from build123d import *

# Parameters (mm, degrees)
SKETCH2_R           = 2.032
BOSS_EXTRUDE1_DEPTH = 3.175


with BuildPart() as part:
    # Sketch2 → Boss-Extrude1 (new, symmetric)
    with BuildSketch(Plane.XY):
        with BuildLine():
            Line((0, 6.35), (231.775, 6.35))
            ThreePointArc((231.775, 6.35), (238.125, 0), (231.775, -6.35))
            Line((231.775, -6.35), (0, -6.35))
            ThreePointArc((0, -6.35), (-6.35, 0), (0, 6.35))
        make_face()
        Circle(SKETCH2_R, mode=Mode.SUBTRACT)
        with Locations((231.775, 0)):
            Circle(SKETCH2_R, mode=Mode.SUBTRACT)
        with Locations((76.2, 0)):
            Circle(SKETCH2_R, mode=Mode.SUBTRACT)
        with Locations((107.95, 0)):
            Circle(SKETCH2_R, mode=Mode.SUBTRACT)
    extrude(amount=BOSS_EXTRUDE1_DEPTH, both=True)


solid = part.part
Work out the finished part from the listing and answer in its coordinate system (mm). Round coordinates to 2 decimals unless told otherwise and drop trailing zeros. Write each loop counter-clockwise with the first axis right and the second up, starting at its lowest first coordinate (ties: lowest second). Pieces come first, ordered by that corner, then holes. Notation, with made-up numbers: (29.25, 42) -> (83.25, 42) arc R17 ccw to (83.25, 68) -> close; hole circle Ø8 at (-37, -15.5). An arc over 180 degrees is marked (long way). Answer as CSV lines item,"result". Start each with the question number.
(1) Find the intervals of material crossed by probe 1 along Y at (x, z) = (107.95, -1.5); probe 2 along X at (y, z) = (1.75, -0.25), in increasing order.
(2) The mould has two halves that part along X. Classify faces 1 (the flat face through (118, 0, -3.175)), 2 (the cylindrical face through (233.65, -0.78, -0.04)), 3 (the cylindrical face through (-0.44, -1.984, -0.044)), 4 (the cylindrical face through (-6.35, -0.14, 0.04)): +X half, -X half, draft (parallel to the pull), parting line (faces both ways), or undercut.
(3) The part is cut by section C-C, the plane z = 0.25. Give the vertices of the cut face in (x, y) (3 decimals).
(4) Each of these flat-tipped pins is pushed along its axis until it touches: pin 1 (3.5 mm diameter, centred on x = 76.2, y = 0, fed in from +Z); pin 2 (1.5 mm diameter, centred on y = -4.5, z = 1.5, fed in from +X); pin 3 (1 mm diameter, centred on y = -3.5, z = -1.5, fed in from +X). Where does it stop, or does it pass through?
(5) The part is cut by section A-A, the plane y = 0. Give the vertices of the cut face in (x, z) (3 decimals).
(6) The part is cut by section B-B, the plane x = 76.2. Give the vertices of the cut face in (y, z) (3 decimals).
Output values:
1,probe 1,"y = -6.35 to -2.03, 2.03 to 6.35"
1,probe 2,"x = -6.1 to -1.03, 1.03 to 75.17, 77.23 to 106.92, 108.98 to 230.74, 232.81 to 237.88"
2,face 1,"draft"
2,face 2,"undercut"
2,face 3,"undercut"
2,face 4,"-X half"
3,outline,"(0, -6.35) -> (231.775, -6.35) arc R6.35 ccw to (231.775, 6.35) -> (0, 6.35) arc R6.35 ccw to start; hole circle Ø4.064 at (0, 0); hole circle Ø4.064 at (76.2, 0); hole circle Ø4.064 at (107.95, 0); hole circle Ø4.064 at (231.775, 0)"
4,pin 1,"passes through"
4,pin 2,"stops at x = 236.9"
4,pin 3,"stops at x = 237.37"
5,outline,"(-6.35, -3.175) -> (-2.032, -3.175) -> (-2.032, 3.175) -> (-6.35, 3.175) -> close; (2.032, -3.175) -> (74.168, -3.175) -> (74.168, 3.175) -> (2.032, 3.175) -> close; (78.232, -3.175) -> (105.918, -3.175) -> (105.918, 3.175) -> (78.232, 3.175) -> close; (109.982, -3.175) -> (229.743, -3.175) -> (229.743, 3.175) -> (109.982, 3.175) -> close; (233.807, -3.175) -> (238.125, -3.175) -> (238.125, 3.175) -> (233.807, 3.175) -> close"
6,outline,"(-6.35, -3.175) -> (-2.032, -3.175) -> (-2.032, 3.175) -> (-6.35, 3.175) -> close; (2.032, -3.175) -> (6.35, -3.175) -> (6.35, 3.175) -> (2.032, 3.175) -> close"
